from build123d import *

# Parameters (mm, degrees)
IZIM1_R                     = 6
Y_KSEKLIK_EKSTR_ZYON1_DEPTH = 4
IZIM2_R                     = 8.5
Y_KSEKLIK_EKSTR_ZYON2_DEPTH = 2
RADYUS1_R                   = 1
IZIM3_R                     = 7.5
Y_KSEKLIK_EKSTR_ZYON3_DEPTH = 17
IZIM4_W                     = 0.657456129
IZIM4_H                     = 1.607114982
IZIM4_W_2                   = 0.693981469
IZIM4_H_2                   = 1.369700268
Y_KSEKLIK_EKSTR_ZYON4_DEPTH = 7


with BuildPart() as part:
    # Çizim1 → Yükseklik-Ekstrüzyon1 (new body)
    with BuildSketch(Plane(origin=(0, 0, 0), x_dir=(1, 0, 0), z_dir=(0, 1, 0))):
        Circle(IZIM1_R)
    extrude(amount=Y_KSEKLIK_EKSTR_ZYON1_DEPTH)

    # Çizim2 → Yükseklik-Ekstrüzyon2 (add)
    with BuildSketch(Plane.XZ):
        Circle(IZIM2_R)
    extrude(amount=Y_KSEKLIK_EKSTR_ZYON2_DEPTH)

    # Radyus1
    radyus1_edges = [part.edges().sort_by_distance(p)[0] for p in [
        (-8.5, 0, 0),
        (-6, 0, 0),
    ]]
    fillet(radyus1_edges, radius=RADYUS1_R)

    # Çizim3 → Yükseklik-Ekstrüzyon3 (add)
    with BuildSketch(Plane.XZ.offset(2)):
        Circle(IZIM3_R)
    extrude(amount=Y_KSEKLIK_EKSTR_ZYON3_DEPTH)

    # Çizim4 → Yükseklik-Ekstrüzyon4 (add)
    with BuildSketch(Plane.XZ.offset(19)):
        with Locations((3.360331326, 3.926474103)):
            Rectangle(IZIM4_W, IZIM4_H)
        with Locations((0.091313352, 3.926474103)):
            Rectangle(IZIM4_W_2, IZIM4_H)
        with Locations((3.360331326, 0.684850134)):
            Rectangle(IZIM4_W, IZIM4_H_2)
        with Locations((0.091313352, 0.684850134)):
            Rectangle(IZIM4_W_2, IZIM4_H_2)
    extrude(amount=Y_KSEKLIK_EKSTR_ZYON4_DEPTH)


solid = part.part
The model under review builds one solid part; all positions refer to its coordinate system, in mm. A direction names the side the tool comes from. Give positions to 0.01 mm unless a question says otherwise; leave off trailing zeros. Order: outer loops, then holes, each group sorted by start corner. A loop starts at its lowest first (then second) coordinate and runs counter-clockwise, first axis right, second up. Notation, with made-up numbers: M -16.75,-11 L -8.75,-11 A8 ccw -8.75,2 Z; hole C -24,-12.75 d8. An arc over 180 degrees is marked long. Use one line per item in the form item = value. Start each with the question number.
Item 1: The part is to be moulded in two halves that separate along X. For faces 1 (the cylindrical face through (4.57, -1.493, 7.167)), 2 (the flat face through (3.032, -22, 1)), 3 (the flat face through (-2, 0, -7)), say which applies: pulls with the +X half, pulls with the -X half, needs draft (parallel to the pull), parting line crosses it, or undercut.
Item 2: To check wall thickness, follow line 1 along Y through (x, z) = (-0.75, 1); line 2 along Y through (x, z) = (-2.5, 6.75); line 3 along Z through (x, y) = (4.5, -4.5). State the ranges of each line that lie inside material, in increasing order. Write a range as from..to.
Item 3: For faces 4 (the cylindrical face through (-7.493, -10.381, 0.33)), 5 (the flat face through (3.689, -22, 4)), 6 (the flat face through (0.438, -22, 4)), 7 (the flat face through (-0.256, -22, 4)), 8 (the cylindrical face through (-6, 2, 0)), list the 3-axis set-ups (+Z, -Z, +X, -X, +Y, -Y) from which the entire face can be reached by the end or side of a thin tool; tool diameter is ignored.
Item 4: We need section B-B on y = -8.25. Give the boundary of the cut face in (x, z).
Item 5: Insertion check: pin 1 Ø5 at (x, y) = (1.5, -22.5) entering from -Z; pin 2 Ø2 at (x, y) = (-5, -7.5) entering from -Z; pin 3 Ø0.5 at (x, y) = (3, -23.5) entering from +Z. Each pin has a flat end and moves straight along its axis. Give the tip position at first contact, or say it passes through.
Item 6: We need section A-A on y = -21.75. Give the boundary of the cut face in (x, z), plus the area to 3 significant figures.
Completed:
q1.face_1 = parting line crosses it
q1.face_2 = undercut
q1.face_3 = needs draft
q2.line_1 = -19..4
q2.line_2 = -19..0
q2.line_3 = -6..6
q3.face_4 = -Y
q3.face_5 = +Z, -Z, +X, -Y
q3.face_6 = +Z, -Z, -Y
q3.face_7 = +Z, -Z, -X, -Y
q3.face_8 = +Y
q4.outline = C 0,0 d15
q5.pin_1 = 0
q5.pin_2 = -6.34
q5.pin_3 = 4.73
q6.outline = M -0.26,0 L 0.44,0 L 0.44,1.37 L -0.26,1.37 Z; M -0.26,3.12 L 0.44,3.12 L 0.44,4.73 L -0.26,4.73 Z; M 3.03,0 L 3.69,0 L 3.69,1.37 L 3.03,1.37 Z; M 3.03,3.12 L 3.69,3.12 L 3.69,4.73 L 3.03,4.73 Z
q6.area = 4.02 mm²
